Check sheet for the modelled part. Datum: model origin and axes. Units: mm. A direction names the side the tool comes from. Round coordinates to 2 decimals unless told otherwise and drop trailing zeros. Order: outer loops, then holes, each group sorted by start corner. A loop starts at its lowest first (then second) coordinate and runs counter-clockwise, first axis right, second up. Notation, with made-up numbers: (74, 32) -> (122, 32) arc R9 cw to (122, 47) -> close; hole circle Ø1 at (-27.75, 84). An arc over 180 degrees is marked (long way). Use CSV: the item, a comma, the result in double quotes.
```python
from build123d import *

# Parameters (mm, degrees)
ESQUISSE1_W             = 10
ESQUISSE1_H             = 10
BOSS_EXTRU_1_DEPTH      = 39
ESQUISSE2_W             = 10
ESQUISSE2_H             = 5
ENL_V_MAT_EXTRU_1_DEPTH = 10
ESQUISSE3_R             = 1.5
ENL_V_MAT_EXTRU_2_DEPTH = 10
ESQUISSE4_R             = 1.5
ENL_V_MAT_EXTRU_3_DEPTH = 42.484937025
ESQUISSE5_R             = 1.5
ENL_V_MAT_EXTRU_4_DEPTH = 42.484937025
ESQUISSE6_R             = 1.5
ENL_V_MAT_EXTRU_5_DEPTH = 42.484937025


with BuildPart() as part:
    # Esquisse1 → Boss.-Extru.1 (new body)
    with BuildSketch(Plane.XY):
        with Locations((5, 5)):
            Rectangle(ESQUISSE1_W, ESQUISSE1_H)
    extrude(amount=BOSS_EXTRU_1_DEPTH)

    # Esquisse2 → Enlèv. mat.-Extru.1 (cut)
    with BuildSketch(Plane.ZY):
        with Locations((34, 2.5)):
            Rectangle(ESQUISSE2_W, ESQUISSE2_H)
    extrude(amount=-ENL_V_MAT_EXTRU_1_DEPTH, mode=Mode.SUBTRACT)

    # Esquisse3 → Enlèv. mat.-Extru.2 (cut)
    with BuildSketch(Plane(origin=(0, 0, 0), x_dir=(-1, 0, 0), z_dir=(0, 0, -1))):
        with Locations((-5, 5)):
            Circle(ESQUISSE3_R)
    extrude(amount=-ENL_V_MAT_EXTRU_2_DEPTH, mode=Mode.SUBTRACT)

    # Esquisse4 → Enlèv. mat.-Extru.3 (cut, through all)
    with BuildSketch(Plane(origin=(0, 10, 0), x_dir=(1, 0, 0), z_dir=(0, 1, 0))):
        with Locations(Location((5, -34, 0), (0, 0, 270))):
            Circle(ESQUISSE4_R)
    extrude(amount=-ENL_V_MAT_EXTRU_3_DEPTH, mode=Mode.SUBTRACT)

    # Esquisse5 → Enlèv. mat.-Extru.4 (cut, through all)
    with BuildSketch(Plane.ZY):
        with Locations((19.5, 5)):
            Circle(ESQUISSE5_R)
    extrude(amount=-ENL_V_MAT_EXTRU_4_DEPTH, mode=Mode.SUBTRACT)

    # Esquisse6 → Enlèv. mat.-Extru.5 (cut, through all)
    with BuildSketch(Plane(origin=(0, 10, 0), x_dir=(1, 0, 0), z_dir=(0, 1, 0))):
        with Locations(Location((5, -14.5, 0), (0, 0, 270))):
            Circle(ESQUISSE6_R)
    extrude(amount=-ENL_V_MAT_EXTRU_5_DEPTH, mode=Mode.SUBTRACT)


solid = part.part
```
Q1. Sectioned sample at C-C, the plane z = 7. Enter the section's corners in (x, y), then the cut area to 3 significant figures.
Result sheet:
outline,"(0, 0) -> (10, 0) -> (10, 10) -> (0, 10) -> close; hole circle Ø3 at (5, 5)"
area,"92.9 mm^2"
Q2. Sectioned sample at B-B, the plane y = 4.5. Enter the section's corners in (x, z).
Result sheet:
outline,"(0, 0) -> (3.59, 0) -> (3.59, 10) -> (6.41, 10) -> (6.41, 0) -> (10, 0) -> (10, 18.09) -> (0, 18.09) -> close; (0, 20.91) -> (10, 20.91) -> (10, 29) -> (0, 29) -> close; hole circle Ø3 at (5, 14.5)"
Q3. Mould release check, pull along X, two halves, no side actions. Record for faces 4 (the face through (0, 5, 15)), 5 (the face through (10, 5, 15)), 6 (the face through (3.8, 6.2, 0)), 7 (the face through (4.1, 7.5, 32.8)): pulls with the +X half, pulls with the -X half, needs draft (parallel to the pull), parting line crosses it, or undercut.
Result sheet:
face 4,"pulls with the -X half"
face 5,"pulls with the +X half"
face 6,"needs draft"
face 7,"undercut"
Q4. Go/stop test with flat-tipped pins: pin 1 (1.5 mm diameter, centred on x = 5, y = 5.5, fed in from -Z); pin 2 (5 mm diameter, centred on x = 5, z = 34, fed in from -Y). Record where each tip stops, or that it passes through.
Result sheet:
pin 1,"stops at z = 10"
pin 2,"stops at y = 5"
Q5. Sectioned sample at D-D, the plane z = 19.5. Enter the section's corners in (x, y).
Result sheet:
outline,"(0, 0) -> (10, 0) -> (10, 3.5) -> (0, 3.5) -> close; (0, 6.5) -> (10, 6.5) -> (10, 10) -> (0, 10) -> close"
Q6. Access from +Z, -Z, +X, -X, +Y, -Y to the whole of each face (thin tool, end or side, straight path). Record for faces 1 (the face through (5, 5, 13)), 2 (the face through (3.8, 5, 32.8)), 3 (the face through (6.2, 4.1, 4.9)).
Result sheet:
face 1,"+Y, -Y"
face 2,"+Z, +X, -X, -Y"
face 3,"-Z"
Q7. Scan lines: L1, parallel to Y at x = 5, z = 4.25; L2, parallel to Y at x = 4.75, z = 20. Record each from-to range of solid material in increasing order.
Result sheet:
L1,"y = 0 to 3.5, 6.5 to 10"
L2,"y = 0 to 3.59, 6.41 to 10"
Q8. Sectioned sample at A-A, the plane x = 5. Enter the section's corners in (y, z), then the cut area to 3 significant figures.
Result sheet:
outline,"(0, 0) -> (3.5, 0) -> (3.5, 10) -> (6.5, 10) -> (6.5, 0) -> (10, 0) -> (10, 13) -> (0, 13) -> close; (0, 16) -> (10, 16) -> (10, 32.5) -> (5, 32.5) -> (5, 29) -> (0, 29) -> close; (5, 35.5) -> (10, 35.5) -> (10, 39) -> (5, 39) -> close; hole circle Ø3 at (5, 19.5)"
area,"258 mm^2"
